from build123d import *

# Parameters (mm, degrees)
SKETCH1_R           = 4.572
SKETCH1_R_2         = 4.445
BOSS_EXTRUDE1_DEPTH = 6.731
BOSS_EXTRUDE3_START = -13.208
SKETCH1_5_R         = 4.572
SKETCH1_5_R_2       = 1.2954
SKETCH1_5_R_3       = 4.445
SKETCH1_5_W         = 13.97
SKETCH1_5_H         = 24.765
BOSS_EXTRUDE3_DEPTH = 3.937
SKETCH4_R           = 1.7
CUT_EXTRUDE4_DEPTH  = 3.81
BOSS_EXTRUDE5_DEPTH = 16.4211
BOSS_EXTRUDE6_DEPTH = 4.572


with BuildPart() as part:
    # Sketch1 (on Front Plane) → Boss-Extrude1 (new body)
    with BuildSketch(Plane.XY):
        with BuildLine():
            Line((-12.7, 0), (-9.525, 16.51))
            Line((-9.525, 16.51), (9.525, 16.51))
            Line((9.525, 16.51), (12.7, 0))
            Line((12.7, 0), (12.7, -46.99))
            ThreePointArc((12.7, -46.99), (0, -59.69), (-12.7, -46.99))
            Line((-12.7, -46.99), (-12.7, 0))
        make_face()
        Circle(SKETCH1_R, mode=Mode.SUBTRACT)
        with Locations((0, -46.99)):
            Circle(SKETCH1_R_2, mode=Mode.SUBTRACT)
    extrude(amount=BOSS_EXTRUDE1_DEPTH)

    # Sketch4 → Cut-Extrude4 (cut)
    with BuildSketch(Plane(origin=(0, 0, 0), x_dir=(-1, 0, 0), z_dir=(0, 0, -1))):
        with BuildLine():
            Line((12.7, -14.099075092), (12.7, 0))
            Line((12.7, 0), (11.302104433, 7.269056948))
            Line((11.302104433, 7.269056948), (10.037418608, 13.84542324))
            Line((10.037418608, 13.84542324), (1.021082558, 8.023816422))
            ThreePointArc((1.021082558, 8.023816422), (0, 7.408645479), (-1.021082558, 8.023816422))
            Line((-1.021082558, 8.023816422), (-10.037418608, 13.84542324))
            Line((-10.037418608, 13.84542324), (-11.47556666, 6.367053366))
            Line((-11.47556666, 6.367053366), (-8.023816422, 1.021082558))
            ThreePointArc((-8.023816422, 1.021082558), (-7.408645479, 0), (-8.023816422, -1.021082558))
            Line((-8.023816422, -1.021082558), (-12.7, -8.263420264))
            Line((-12.7, -8.263420264), (-12.7, -14.099075092))
            ThreePointArc((-12.7, -14.099075092), (-11.380658922, -14.323016968), (-10.113003756, -13.894226547))
            Line((-10.113003756, -13.894226547), (-1.021082558, -8.023816422))
            ThreePointArc((-1.021082558, -8.023816422), (0, -7.408645479), (1.021082558, -8.023816422))
            Line((1.021082558, -8.023816422), (10.113003756, -13.894226547))
            ThreePointArc((10.113003756, -13.894226547), (11.380658922, -14.323016968), (12.7, -14.099075092))
        make_face()
        Circle(SKETCH4_R, mode=Mode.SUBTRACT)
    extrude(amount=-CUT_EXTRUDE4_DEPTH, mode=Mode.SUBTRACT)



with BuildPart() as body_2:
    # Sketch1<5> → Boss-Extrude3 (new body)
    with BuildSketch(Plane.XY.offset(BOSS_EXTRUDE3_START)):
        with BuildLine():
            Line((-12.7, 0), (-9.525, 16.51))
            Line((-9.525, 16.51), (9.525, 16.51))
            Line((9.525, 16.51), (12.7, 0))
            Line((12.7, 0), (12.7, -46.99))
            ThreePointArc((12.7, -46.99), (0, -59.69), (-12.7, -46.99))
            Line((-12.7, -46.99), (-12.7, 0))
        make_face()
        Circle(SKETCH1_5_R, mode=Mode.SUBTRACT)
        with Locations((0, -10.16)):
            Circle(SKETCH1_5_R_2, mode=Mode.SUBTRACT)
        with Locations((0, -38.1)):
            Circle(SKETCH1_5_R_2, mode=Mode.SUBTRACT)
        with Locations((0, -46.99)):
            Circle(SKETCH1_5_R_3, mode=Mode.SUBTRACT)
        with Locations((0, -24.13)):
            Rectangle(SKETCH1_5_W, SKETCH1_5_H, mode=Mode.SUBTRACT)
    extrude(amount=-BOSS_EXTRUDE3_DEPTH)


with BuildPart() as part_1:
    add(part.part)

    add(body_2.part)  # Boss-Extrude5 merges body 2
    # Sketch5 → Boss-Extrude5 (add)
    with BuildSketch(Plane(origin=(0, 0, 0), x_dir=(-1, 0, 0), z_dir=(0, 0, -1))):
        Polygon((-9.525, 16.51), (9.525, 16.51), (10.282115385, 12.573), (-10.282115385, 12.573), align=None)
    extrude(amount=BOSS_EXTRUDE5_DEPTH)

    # Sketch4<3> → Boss-Extrude6 (add)
    with BuildSketch(Plane(origin=(0, 0, 0), x_dir=(-1, 0, 0), z_dir=(0, 0, -1))):
        with BuildLine():
            Line((11.47556666, 6.367053366), (8.023816422, 1.021082558))
            ThreePointArc((8.023816422, 1.021082558), (7.408645479, 0), (8.023816422, -1.021082558))
            Line((8.023816422, -1.021082558), (12.7, -8.263420264))
            Line((12.7, -8.263420264), (12.7, 0))
            Line((12.7, 0), (11.47556666, 6.367053366))
        make_face()
    extrude(amount=-BOSS_EXTRUDE6_DEPTH)


solid = part_1.part
Part model, mm, in its own coordinate system. A direction names the side the tool comes from. Coordinates: 2 decimals unless noted, no trailing zeros. Loops run counter-clockwise (first coordinate to the right, second up) from the corner with the lowest first, then second, coordinate; pieces in that order, holes last. Notation, with made-up numbers: (73, 74) -> (88, 74) arc R17 ccw to (88, 99) -> close; hole circle Ø7 at (-28.75, -22.5). An arc over 180 degrees is marked (long way). Use a Markdown table: item, result. Add a question column.
Item 1: Which spindle directions (+Z, -Z, +X, -X, +Y, -Y) get a long thin tool onto all of the face, cutting with end or side? Do faces 1 (the flat face through (10.33, -4.59, 1.88)), 2 (the flat face through (0, 12.573, -7)), 3 (the flat face through (9.4, 12.9, 0)). Say none if no direction does.
Item 2: Flat gauge pins, fed straight in: P1, Ø1.5, axis at x = 5, z = -6.5, coming from the -Y side; P2, Ø8, axis at x = 0, y = 0, coming from the +Z side; P3, Ø4, axis at y = 8.5, z = -11.5, coming from the -X side; P4, Ø3, axis at y = 4.5, z = -1, coming from the +X side. Where does each tip first touch, or does it go through?
Item 3: Band-saw the part on D-D on x = 2.5. Give the number of separate pieces and of enclosed holes in the cut face, plus the area to 3 significant figures.
Item 4: Band-saw the part on A-A on z = 2.5. Write the cut outline in (x, y) (3 decimals).
Item 5: Band-saw the part on B-B on y = -38.1. Write the cut outline in (x, z) (3 decimals).
Item 6: Pull direction Y, two halves, no side cores. Call faces 4 (the flat face through (0, 16.51, -5)), 5 (the flat face through (-8, -23, -13.208)), 6 (the cylindrical face through (7.41, 0.02, 1.88)), 7 (the flat face through (-9.774, 3.731, 1.878)): +Y half, -Y half, draft (parallel to the pull), parting line (faces both ways), or undercut.
Item 7: Band-saw the part on C-C on y = -48.5. Write the cut outline in (x, z) (3 decimals), plus the area to 3 significant figures.
Item 8: Probe probe 1 along Y at (x, z) = (0, 5.5) (3 decimals); probe 2 along Z at (x, y) = (5.5, 11) (3 decimals); probe 3 along Y at (x, z) = (0, -14.35) (1 decimal). List the from-to ranges inside material, lowest first.
Geometry says:
| question | item | result |
|---|---|---|
| 1 | face 1 | none |
| 1 | face 2 | +X, -X, -Y |
| 1 | face 3 | +X |
| 2 | P1 | y = 12.57 |
| 2 | P2 | through |
| 2 | P3 | x = -11.27 |
| 2 | P4 | x = 12.05 |
| 3 | separate pieces | 6 |
| 3 | enclosed holes | 0 |
| 3 | area | 565 mm² |
| 4 | outline | (-12.7, -46.99) arc R12.7 ccw to (12.7, -46.99) -> (12.7, -14.099) arc R2.735 cw to (10.113, -13.894) -> (1.021, -8.024) arc R1.155 ccw to (-1.021, -8.024) -> (-10.113, -13.894) arc R2.735 cw to (-12.7, -14.099) -> close; (-12.7, -8.263) -> (-8.024, -1.021) arc R1.155 ccw to (-8.024, 1.021) -> (-11.476, 6.367) -> (-12.7, 0) -> close; (-10.037, 13.845) -> (-1.021, 8.024) arc R1.155 ccw to (1.021, 8.024) -> (10.037, 13.845) -> (9.525, 16.51) -> (-9.525, 16.51) -> close; (8.024, -1.021) -> (12.7, -8.263) -> (12.7, 0) -> (11.476, 6.367) -> (8.024, 1.021) arc R1.155 ccw to start; hole circle Ø8.89 at (0, -46.99) |
| 5 | outline | (-12.7, -17.145) -> (-1.295, -17.145) -> (-1.295, -13.208) -> (-12.7, -13.208) -> close; (-12.7, 0) -> (12.7, 0) -> (12.7, 6.731) -> (-12.7, 6.731) -> close; (1.295, -17.145) -> (12.7, -17.145) -> (12.7, -13.208) -> (1.295, -13.208) -> close |
| 6 | face 4 | +Y half |
| 6 | face 5 | draft |
| 6 | face 6 | undercut |
| 6 | face 7 | undercut |
| 7 | outline | (-12.61, -17.145) -> (-4.181, -17.145) -> (-4.181, -13.208) -> (-12.61, -13.208) -> close; (-12.61, 0) -> (-4.181, 0) -> (-4.181, 6.731) -> (-12.61, 6.731) -> close; (4.181, -17.145) -> (12.61, -17.145) -> (12.61, -13.208) -> (4.181, -13.208) -> close; (4.181, 0) -> (12.61, 0) -> (12.61, 6.731) -> (4.181, 6.731) -> close |
| 7 | area | 180 mm² |
| 8 | probe 1 | -59.69 to -51.435, -42.545 to -4.572, 4.572 to 16.51 |
| 8 | probe 2 | -17.145 to -13.208, 0 to 6.731 |
| 8 | probe 3 | -59.7 to -51.4, -42.5 to -39.4, -36.8 to -36.5, -11.7 to -11.5, -8.9 to -4.6, 4.6 to 16.5 |
